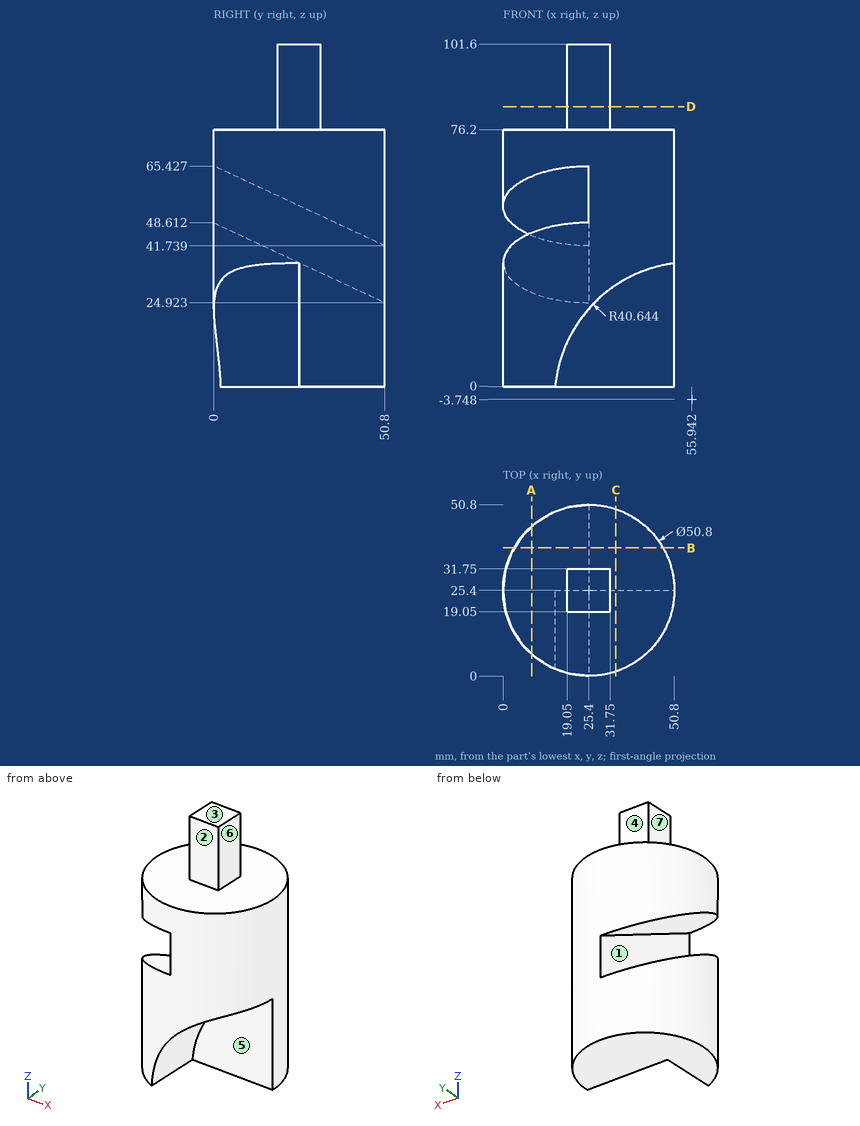
Verification items for this drawing (mm, ordinates from the low corner). A direction names the side the tool comes from. Give positions to 0.01 mm unless a question says otherwise; leave off trailing zeros. Write each loop counter-clockwise with the first axis right and the second up, starting at its lowest first coordinate (ties: lowest second). Pieces come first, ordered by that corner, then holes. Notation, with made-up numbers: (5, 22) -> (43, 22) arc R17 cw to (43, 47) -> close; hole circle Ø3 at (-26, 28). An arc over 180 degrees is marked (long way). Use CSV: the item, a comma, the result in double quotes. Start each with the question number.
Q1. Scan lines: line 1 along Z through (x, y) = (46.5, 27.5); line 2 along X through (y, z) = (24, 83.5); line 3 along Z through (x, y) = (6.5, 37) (1 decimal). Record each from-to range of solid material in increasing order.
Q2. Tool access check on the marked faces 4, 5, 6 and 7. Record the directions out of +Z, -Z, +X, -X, +Y, -Y that give a thin tool (end or side, any length) a straight path to the whole face; none if there is none.
Q3. Depth check by flat-ended pin: P1, Ø14, axis at y = 27, z = 84.5, coming from the +X side; P2, Ø12, axis at y = 35.5, z = 38, coming from the -X side; P3, Ø4, axis at x = 26.5, z = 90, coming from the +Y side. Enter the tip coordinate at first touch or a pass-through.
Q4. Release check for a two-part mould opening along Z. For the marked faces 1, 2 and 3 record: +Z half, -Z half, draft (parallel to the pull), parting line (faces both ways), or undercut.
Q5. Cross-section at A-A on x = 8.5. Enter the section's corners in (y, z) (1 decimal), and give its area (3 significant figures).
Q6. Cross-section at C-C on x = 33.5. Enter the section's corners in (y, z).
Q7. Cross-section at D-D on z = 83. Enter the section's corners in (x, y), and give its area (3 significant figures).
Q8. Cross-section at B-B on y = 38. Enter the section's corners in (x, z) (1 decimal), and give its area (3 significant figures).
Working result:
1,line 1,"z = 0 to 76.2"
1,line 2,"x = 19.05 to 31.75"
1,line 3,"z = 0 to 31.4, 48.2 to 76.2"
2,face 4,"+Z, +X, -X, +Y"
2,face 5,"-Z, +X, -Y"
2,face 6,"+Z, +X, +Y, -Y"
2,face 7,"+Z, -X, +Y, -Y"
3,P1,"stops at x = 31.75"
3,P2,"stops at x = 0.59"
3,P3,"stops at y = 31.75"
4,face 1,"undercut"
4,face 2,"draft"
4,face 3,"+Z half"
5,outline,"(6.4, 0) -> (44.4, 0) -> (44.4, 27.9) -> (6.4, 45.6) -> close; (6.4, 62.4) -> (44.4, 44.7) -> (44.4, 76.2) -> (6.4, 76.2) -> close"
5,area,"2,250 mm^2"
6,outline,"(1.33, 30.14) -> (25.4, 30.14) -> (25.4, 0) -> (49.47, 0) -> (49.47, 76.2) -> (1.33, 76.2) -> close"
7,outline,"(19.05, 19.05) -> (31.75, 19.05) -> (31.75, 31.75) -> (19.05, 31.75) -> close"
7,area,"161 mm^2"
8,outline,"(3.3, 0) -> (47.5, 0) -> (47.5, 76.2) -> (3.3, 76.2) -> (3.3, 47.7) -> (25.4, 47.7) -> (25.4, 30.9) -> (3.3, 30.9) -> close"
8,area,"2,990 mm^2"
